```python
from build123d import *

# Parameters (mm, degrees)
SKETCH1_W            = 84
SKETCH1_H            = 60
BOSS_EXTRUDE1_DEPTH  = 2.85
SKETCH2_W            = 3
SKETCH2_H            = 15
CUT_EXTRUDE1_DEPTH   = 52.692576837
CUT_EXTRUDE2_DEPTH   = 52.692576837
SKETCH4_W            = 10
SKETCH4_H            = 2.85
BOSS_EXTRUDE2_DEPTH  = 2.85
MIRROR3_COPY_1_DEPTH = 52.692576837
SKETCH5_R            = 1.7
CUT_EXTRUDE3_DEPTH   = 6


with BuildPart() as part:
    # Sketch1 → Boss-Extrude1 (new body)
    with BuildSketch(Plane(origin=(0, 0, 0), x_dir=(1, 0, 0), z_dir=(0, 1, 0))):
        Rectangle(SKETCH1_W, SKETCH1_H)
    extrude(amount=BOSS_EXTRUDE1_DEPTH)

    # Sketch2 → Cut-Extrude1 (cut, through all)
    with BuildSketch(Plane.XZ):
        with Locations((-34.4, 22.5)):
            Rectangle(SKETCH2_W, SKETCH2_H)
    cut_extrude1 = extrude(amount=-CUT_EXTRUDE1_DEPTH, mode=Mode.SUBTRACT)

    # Mirror1: Cut-Extrude1 across plane
    add(cut_extrude1.mirror(Plane(origin=(0, 0, 0), x_dir=(0, 0, 1), z_dir=(1, 0, 0))), mode=Mode.SUBTRACT)

    # Sketch3 → Cut-Extrude2 (cut, through all)
    with BuildSketch(Plane(origin=(0, 2.85, 0), x_dir=(1, 0, 0), z_dir=(0, 1, 0))):
        Polygon((-23.3, 26), (-21, 26), (-21, 30), (-17.6, 30), (-17.6, 26), (-15.3, 26), (-15.3, 23), (-17.6, 23), (-17.6, 20), (-21, 20), (-21, 23), (-23.3, 23), align=None)
    cut_extrude2 = extrude(amount=-CUT_EXTRUDE2_DEPTH, mode=Mode.SUBTRACT)

    # Mirror2: Cut-Extrude2 across plane
    add(cut_extrude2.mirror(Plane(origin=(0, 0, 0), x_dir=(0, 0, 1), z_dir=(1, 0, 0))), mode=Mode.SUBTRACT)

    # Sketch4 → Boss-Extrude2 (add)
    with BuildSketch(Plane(origin=(0, 2.85, 0), x_dir=(1, 0, 0), z_dir=(0, 1, 0))):
        with Locations((0, 31.425)):
            Rectangle(SKETCH4_W, SKETCH4_H)
    boss_extrude2 = extrude(amount=-BOSS_EXTRUDE2_DEPTH)

    # Mirror3: Cut-Extrude2, Boss-Extrude2 across plane
    add(cut_extrude2.mirror(Plane.XY), mode=Mode.SUBTRACT)
    add(boss_extrude2.mirror(Plane.XY))

    # Mirror3 copy 1 sketch → Mirror3 copy 1 (cut, through all)
    with BuildSketch(Plane(origin=(0, 2.85, 0), x_dir=(-1, 0, 0), z_dir=(0, 1, 0))):
        Polygon((-23.3, 26), (-21, 26), (-21, 30), (-17.6, 30), (-17.6, 26), (-15.3, 26), (-15.3, 23), (-17.6, 23), (-17.6, 20), (-21, 20), (-21, 23), (-23.3, 23), align=None)
    extrude(amount=-MIRROR3_COPY_1_DEPTH, mode=Mode.SUBTRACT)

    # Sketch5 → Cut-Extrude3 (cut)
    with BuildSketch(Plane(origin=(0, 5.35, 32.85), x_dir=(1, 0, 0), z_dir=(0, 1, 0))):
        with Locations(Location((-28.4, 13.35, 0), (0, 0, 270))):
            Circle(SKETCH5_R)
    cut_extrude3 = extrude(amount=-CUT_EXTRUDE3_DEPTH, mode=Mode.SUBTRACT)

    # Mirror4: Cut-Extrude3 across plane
    add(cut_extrude3.mirror(Plane(origin=(0, 0, 0), x_dir=(0, 0, 1), z_dir=(1, 0, 0))), mode=Mode.SUBTRACT)


solid = part.part
```
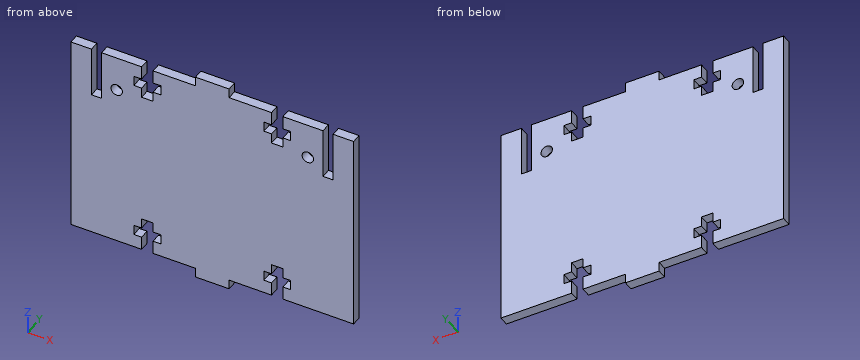
Design review of the part built by this model. Coordinates are the model's own, in mm. Coordinates: 2 decimals unless noted, no trailing zeros. Order: outer loops, then holes, each group sorted by start corner. A loop starts at its lowest first (then second) coordinate and runs counter-clockwise, first axis right, second up. Notation, with made-up numbers: (-1, -4.75) - (30, -4.75) arc R19 cw to (30, 28.25) - close; hole circle Ø1 at (81.25, -36). An arc over 180 degrees is marked (long way). One line per question, with ' | ' between items.
Q1. Consider section A-A, the plane x = -28.4. Give the boundary of the cut face in (y, z), then the cut area to 3 significant figures.
Answer key:
outline: (0, -30) - (2.85, -30) - (2.85, 17.8) - (0, 17.8) - close; (0, 21.2) - (2.85, 21.2) - (2.85, 30) - (0, 30) - close | area: 161 mm2
Q2. Clearance check with flat-ended pins moving along their axes: pin 1 Ø8 at (x, z) = (13.5, 12.5) entering from -Y; pin 2 Ø1.4 at (x, y) = (-39.5, 2) entering from +Z; pin 3 Ø0.7 at (x, y) = (-21.5, 2) entering from -Z. State where each tip first meets the part, or that it passes through.
Answer key:
pin 1: stops at y = 0 | pin 2: stops at z = 30 | pin 3: stops at z = -30
Q3. Consider section B-B, the plane y = 1.55. Give the number of separate pieces and of enclosed holes in the cut face, then the cut area to 3 significant figures.
Answer key:
separate pieces: 1 | enclosed holes: 2 | area: 4,800 mm2
Q4. To check wall thickness, follow line 1 along X through (y, z) = (2.1, 19.5); line 2 along X through (y, z) = (0.3, -29); line 3 along X through (y, z) = (2.25, 21.5). State the ranges of each line that lie inside material, in increasing order.
Answer key:
line 1: x = -42 to -35.9, -32.9 to -30.1, -26.7 to 26.7, 30.1 to 32.9, 35.9 to 42 | line 2: x = -42 to -21, -17.6 to 17.6, 21 to 42 | line 3: x = -42 to -35.9, -32.9 to -21, -17.6 to 17.6, 21 to 32.9, 35.9 to 42
